The figure shows three views and two pictorial views of one solid part (mm, origin at its lowest corner). Answer the questions. A direction names the side the tool comes from. Coordinates: 2 decimals unless noted, no trailing zeros. Loops run counter-clockwise (first coordinate to the right, second up) from the corner with the lowest first, then second, coordinate; pieces in that order, holes last. Notation, with made-up numbers: M 43.25,-13 L 71.25,-13 A19 ccw 71.25,20 Z; hole C -0.75,43 d4. An arc over 180 degrees is marked long. Return JSON: item names as keys, results as strings. Group by question number.
1. Given P1, Ø8, axis at y = 13, z = 33.5, coming from the -X side; P2, Ø1.5, axis at y = 11, z = 43.5, coming from the -X side; P3, Ø6, axis at x = 59.5, y = 17, coming from the -Z side, each flat-ended and moving along its own axis, determine where each tip first touches the part or whether it passes through.
2. Section B-B (x = 90) is taken. Write down the section's boundary in (y, z).
3. Which of the six approach directions +Z, -Z, +X, -X, +Y, -Y give full straight-line access (tool end or side, diameter ignored) to the marked faces 4 and 5?
4. Section D-D (y = 11) is taken. Write down the section's boundary in (x, z).
5. The mould has two halves that part along Z. Classify the marked faces 1, 2 and 3: pulls with the +Z half, pulls with the -Z half, needs draft (parallel to the pull), parting line crosses it, or undercut.
6. Section A-A (z = 47.5) is taken. Write down the section's boundary in (x, y).
7. Straight lines are drawn through the part: L1, parallel to X at y = 26.25, z = 39; L2, parallel to Z at x = 60.5, y = 22.75; L3, parallel to Y at x = 20.5, z = 13.5. For each, find the intervals that lie inside material, in ascending order. Write a range as from..to.
8. Section C-C (z = 112.4) is taken. Write down the section's boundary in (x, y), then the cut area to 3 significant figures.
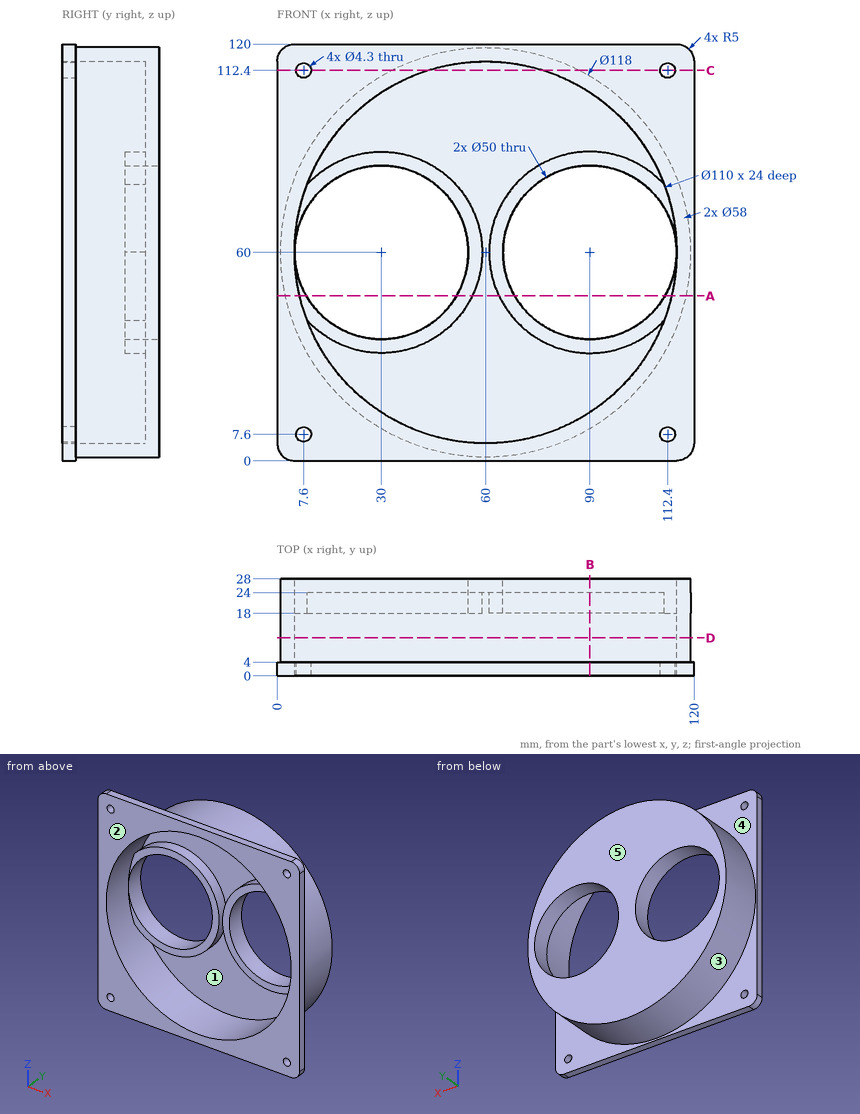
Worked out:
{
 "1": {"P1": "x = 5.46", "P2": "x = 3.14", "P3": "z = 1"},
 "2": {"outline": "M 0,0 L 4,0 L 4,9.2 L 28,9.2 L 28,35 L 18,35 L 18,31 L 24,31 L 24,13.9 L 0,13.9 Z; M 0,106.1 L 24,106.1 L 24,89 L 18,89 L 18,85 L 28,85 L 28,110.8 L 4,110.8 L 4,120 L 0,120 Z"},
 "3": {"face 4": "+Y", "face 5": "+Z, -Z, +X, -X, +Y"},
 "4": {"outline": "C 60,60 d118; hole C 60,60 d110"},
 "5": {"face 1": "undercut", "face 2": "needs draft", "face 3": "parting line crosses it"},
 "6": {"outline": "M 0,0 L 6.44,0 L 6.44,18 L 8.35,18 L 8.35,28 L 2.34,28 L 2.34,4 L 0,4 Z; M 51.65,18 L 56.17,18 L 56.17,24 L 63.83,24 L 63.83,18 L 68.35,18 L 68.35,28 L 51.65,28 Z; M 111.65,18 L 113.56,18 L 113.56,0 L 120,0 L 120,4 L 117.66,4 L 117.66,28 L 111.65,28 Z"},
 "7": {"L1": "4.86..16.44, 43.56..76.44, 103.56..115.14", "L2": "1..5, 115..119", "L3": "0..4"},
 "8": {"outline": "M 0,0 L 5.45,0 L 5.45,4 L 0,4 Z; M 9.75,0 L 43.29,0 L 43.29,24 L 76.71,24 L 76.71,0 L 110.25,0 L 110.25,4 L 87.12,4 L 87.12,28 L 32.88,28 L 32.88,4 L 9.75,4 Z; M 114.55,0 L 120,0 L 120,4 L 114.55,4 Z", "area": "945 mm^2"}
}
